The listing builds one solid part. Answer for the finished solid, in the listing's coordinates (mm). A direction names the side the tool comes from. Give positions to 0.01 mm unless a question says otherwise; leave off trailing zeros. Write each loop counter-clockwise with the first axis right and the second up, starting at its lowest first coordinate (ties: lowest second). Pieces come first, ordered by that corner, then holes. Notation, with made-up numbers: (-18, -15.5) -> (20, -15.5) arc R32 cw to (20, 22.5) -> close; hole circle Ø3 at (17.25, 1). An arc over 180 degrees is marked (long way). One line per question, with ' | ' between items.
Autodesk Inventor part; units mm, degrees
ref_plane "Work Plane1" through (0, -3.975, 0) normal (0, 1, 0) x (-1, 0, 0)
ref_plane "Work Plane2" through (0, 0, 37.3) normal (0, 0, -1) x (-1, 0, 0)
ref_plane "YZ Plane" through (0, 0, 0) normal (1, 0, 0) x (0, 1, 0)
sketch "Sketch1" plane through (0, 0, 0) normal (0, 0, 1) x (1, 0, 0)
  circle A0 centre (0, 0) radius 3.975
  circle A1 centre (0, 0) radius 3.375
  dimension "d0" = 7.95
  dimension "d1" = 0.6
extrude "Extrusion1" add sketch "Sketch1" along normal blind 39.55
ref_plane "Work Plane1" through (0, -3.975, 0) normal (0, 1, 0) x (-1, 0, 0)
sketch "Sketch2" plane through (0, -3.975, 0) normal (0, 1, 0) x (-1, 0, 0)
  line L0 (0, 0) -> (0, 6.8) construction
  line L1 (0, 6.8) -> (0, 32.8) construction
  circle A0 centre (0, 32.8) radius 2.5
  circle A1 centre (0, 6.8) radius 2.5
  line L2 (2.075, 32.8) -> (-2.075, 32.8)
  line L3 (-2.075, 32.8) -> (-2.075, 6.8)
  line L4 (-2.075, 6.8) -> (2.075, 6.8)
  line L5 (2.075, 6.8) -> (2.075, 32.8)
  dimension "d4" = 6.8
  dimension "d5" = 26
  dimension "d6" = 5
  dimension "d7" = 4.15
extrude "Extrusion2" cut sketch "Sketch2" along normal up to surface
ref_plane "Work Plane2" through (0, 0, 37.3) normal (0, 0, -1) x (-1, 0, 0)
sketch "Sketch3" plane through (0, 0, 39.55) normal (0, 0, 1) x (1, 0, 0)
  circle A0 centre (0, 0) radius 3.375
  circle A1 centre (0, 0) radius 3.975
  line L0 (2.15, 4.5) -> (2.15, -4.5)
  line L1 (-2.15, -4.5) -> (-2.15, 4.5)
  line L2 (-2.15, 0) -> (2.15, 0) construction
  arc A2 (-2.15, 4.5) -> (-2.15, -4.5) centre (1.8186, 0) ccw
  arc A3 (2.15, -4.5) -> (2.15, 4.5) centre (-1.8186, 0) ccw
  point P0 (0, 0)
  dimension "d20" = 4.3
  dimension "d21" = 9
  dimension "d22" = 6
  dimension "d23" = 6
extrude "Extrusion3" cut sketch "Sketch3" against normal up to surface (2.25 mm away) contours A0 L0 | A0 L0 A1 | L1 A0 | A0 L1 A1 | L0 A3 A1 | A1 L1 A2
chamfer "Chamfer1" distance 0.25 distance2 0.75 2 edges at (0, -3.375, 39.55) (0, 3.375, 39.55) measured on face at (1.662, -3.3702, 39.55) measured on face at (1.662, 3.3702, 39.55)
chamfer "Chamfer2" distance 0.375 angle 45 4 edges at (2.15, -2.6016, 38.05) (2.15, 2.6016, 38.05) (-2.15, -2.6016, 38.05) (-2.15, 2.6016, 38.05)
properties part number "308-13" material "Steel, Mild"
Item 1: Determine the mould class of faces 1 (the face through (-0.1, -3.7, 4.3)), 2 (the face through (-0.86, 3.88, 19.5)), 3 (the face through (-3.55, -0.23, 37.3)) for opening direction X: pulls with the +X half, pulls with the -X half, needs draft (parallel to the pull), parting line crosses it, or undercut.
Answers below:
face 1: undercut | face 2: parting line crosses it | face 3: needs draft
Item 2: Find section C-C (z = 36.5). Write down the section's boundary in (x, y) (3 decimals).
Answers below:
outline: circle Ø7.95 at (0, 0); hole circle Ø6.75 at (0, 0)
Item 3: Find section A-A (y = -1.75). Write down the section's boundary in (x, z).
Answers below:
outline: (-3.57, 0) -> (-2.89, 0) -> (-2.89, 37.3) -> (-3.57, 37.3) -> close; (2.89, 0) -> (3.57, 0) -> (3.57, 37.3) -> (2.89, 37.3) -> close
Item 4: A tool of negligible diameter and unlimited length cuts with its end or side. For faces 4 (the face through (0.03, 3.474, 39.097)), 5 (the face through (0, -3.8, 39.55)), 6 (the face through (0.1, -3.7, 35.3)), from which of +Z, -Z, +X, -X, +Y, -Y can it reach the whole face along a straight path? Write none if from no direction.
Answers below:
face 4: +Z | face 5: +Z, +X, -X, +Y, -Y | face 6: -Y
Item 5: Flat-ended cylindrical pins translate along their axes: pin 1 (3 mm diameter, centred on x = -0.5, y = -1, fed in from -Z); pin 2 (1.5 mm diameter, centred on x = 0.5, z = 16, fed in from -Y) (3 decimals); pin 3 (1.7 mm diameter, centred on x = 3.5, y = -1, fed in from +Z); pin 4 (2 mm diameter, centred on x = -3, y = 1, fed in from -Z). Find the tip coordinate at first contact, or state that the pin passes through.
Answers below:
pin 1: through | pin 2: y = 3.135 | pin 3: z = 37.3 | pin 4: z = 0
Item 6: Find section D-D (y = 2). Write down the section's boundary in (x, z).
Answers below:
outline: (-3.44, 0) -> (-2.72, 0) -> (-2.72, 37.3) -> (-3.44, 37.3) -> close; (2.72, 0) -> (3.44, 0) -> (3.44, 37.3) -> (2.72, 37.3) -> close
Item 7: Consider line 1 (X direction, y = 0, z = 24) (3 decimals); line 2 (Y direction, x = 3, z = 15). Determine where each line is inside the solid, lowest interval first. Write a range as [from, to].
Answers below:
line 1: [-3.975, -3.375], [3.375, 3.975] | line 2: [-2.61, -1.55], [1.55, 2.61]
Item 8: Find section B-B (x = 0.75). Count the separate pieces of the cut face and the enclosed holes in it, then the cut area to 3 significant figures.
Answers below:
separate pieces: 3 | enclosed holes: 0 | area: 29.4 mm²
